from build123d import *

# Parameters (mm, degrees)
BOSS_EXTRUDE1_DEPTH = 5
SKETCH2_R           = 26.19375
BOSS_EXTRUDE2_DEPTH = 35


with BuildPart() as part:
    # Sketch1 → Boss-Extrude1 (new body)
    with BuildSketch(Plane.XY):
        Polygon((0, 0), (265, 0), (265, 292), (-239, 292), (-239, 167), (0, 167), align=None)
    extrude(amount=BOSS_EXTRUDE1_DEPTH)

    # Sketch2 → Boss-Extrude2 (add)
    with BuildSketch(Plane.XY.offset(5)):
        with Locations((227.686407853, 257.993451028)):
            Circle(SKETCH2_R)
        with Locations((161.807907248, 257.993451028)):
            Circle(SKETCH2_R)
    extrude(amount=BOSS_EXTRUDE2_DEPTH)


solid = part.part
Geometry: final body of the model. Coordinates: model frame, mm. A direction names the side the tool comes from. Coordinates: 2 decimals unless noted, no trailing zeros. Write each loop counter-clockwise with the first axis right and the second up, starting at its lowest first coordinate (ties: lowest second). Pieces come first, ordered by that corner, then holes. Notation, with made-up numbers: (28.25, -2.5) - (82.25, -2.5) arc R14 cw to (82.25, 24.5) - close; hole circle Ø4 at (-21.75, 10.5). An arc over 180 degrees is marked (long way). Return JSON: item names as keys, results as strings.
Item 1: Section query A-A (x = 177). Output: boundary loops of the cut face in (y, z).
Completed:
{"outline": "(0, 0) - (292, 0) - (292, 5) - (279.33, 5) - (279.33, 40) - (236.66, 40) - (236.66, 5) - (0, 5) - close"}
Item 2: Reachability of faces 3 (the face through (239.773, 234.755, 22.255)), 4 (the face through (227, 258, 40)) from +Z, -Z, +X, -X, +Y, -Y: full face, straight path, thin tool, end or side. Return the list, or none.
Completed:
{"face 3": "+Z", "face 4": "+Z, +X, -X, +Y, -Y"}
Item 3: Pin query (flat end, axial travel): pin 1 Ø12 at (y, z) = (144, 5.5) entering from -X; pin 2 Ø2.5 at (x, z) = (-152.5, 1.5) entering from -Y; pin 3 Ø1 at (x, z) = (176, 14.5) entering from -Y; pin 4 Ø3 at (x, z) = (5.5, 5.5) entering from +Y. Return the tip coordinate at first contact, or that it passes through.
Completed:
{"pin 1": "stops at x = 0", "pin 2": "stops at y = 167", "pin 3": "stops at y = 235.66", "pin 4": "stops at y = 292"}
Item 4: Section query B-B (y = 130.5). Output: boundary loops of the cut face in (x, z), and give its area (4 significant figures).
Completed:
{"outline": "(0, 0) - (265, 0) - (265, 5) - (0, 5) - close", "area": "1,325 mm2"}
Item 5: Pull-direction query (X, two-part tool) for faces 1 (the face through (161, 258, 40)), 2 (the face through (173.895, 234.755, 22.255)); classes: +X half, -X half, draft (parallel to the pull), parting line (faces both ways), or undercut.
Completed:
{"face 1": "draft", "face 2": "undercut"}
Item 6: Section query D-D (y = 214). Output: boundary loops of the cut face in (x, z).
Completed:
{"outline": "(-239, 0) - (265, 0) - (265, 5) - (-239, 5) - close"}
Item 7: Line query: L1, parallel to Z at x = 43, y = 252; L2, parallel to X at y = 84.5, z = 4.5; L3, parallel to X at y = 268.5, z = 11.5. Output: solid intervals per line, ascending.
Completed:
{"L1": "z = 0 to 5", "L2": "x = 0 to 265", "L3": "x = 137.81 to 185.8, 203.69 to 251.68"}
Item 8: Section query C-C (z = 10). Output: boundary loops of the cut face in (x, y), and give its area (3 significant figures).
Completed:
{"outline": "circle Ø52.39 at (161.81, 257.99); circle Ø52.39 at (227.69, 257.99)", "area": "4,310 mm2"}
